Part print with two shaded views. Sizes in mm from the minimum x, y, z corner. Round coordinates to 2 decimals unless told otherwise and drop trailing zeros. Loops run counter-clockwise (first coordinate to the right, second up) from the corner with the lowest first, then second, coordinate; pieces in that order, holes last. Notation, with made-up numbers: M 49.5,48 L 55.5,48 A36 ccw 55.5,82 Z; hole C 40.5,54 d5. An arc over 180 degrees is marked long. Answer as CSV lines item,"result". Start each with the question number.
Item 1: Band-saw the part on C-C (z = 5.5). Give the cut face in (x, y).
Item 2: Band-saw the part on D-D (x = 6). Give the cut face in (y, z), and give its area (3 significant figures).
Item 3: Wall check: line 1 (X direction, y = 9.5, z = 51); line 2 (Z direction, x = 27.5, y = 10.5); line 3 (Y direction, x = 13, z = 11). Give the ranges that are in metal, low to high.
Item 4: Band-saw the part on B-B (y = 43). Give the cut face in (x, z), and give its area (3 significant figures).
Item 5: Mould opens along X. For the marked faces 1, 2 and 3 say: pulls with the +X half, pulls with the -X half, needs draft (parallel to the pull), parting line crosses it, or undercut.
Item 6: Drop flat-ended pins along their axis: pin 1 Ø5 at (x, z) = (12.5, 41.5) entering from -Y; pin 2 Ø6 at (x, y) = (15, 16) entering from -Z; pin 3 Ø3 at (x, z) = (9, 66) entering from -Y. Give the stop position or say it passes through.
Item 7: Band-saw the part on A-A (x = 60.5). Give the cut face in (y, z), and give its area (3 significant figures).
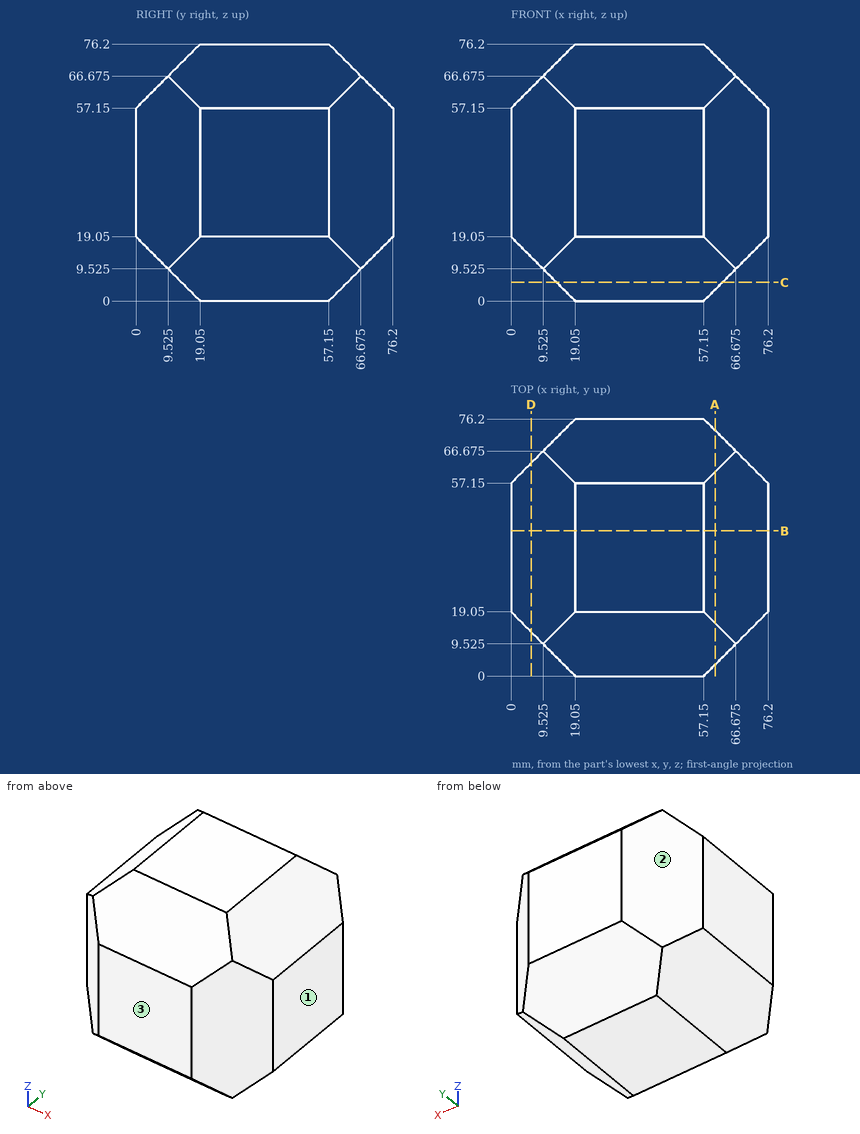
Answer block:
1,outline,"M 13.55,13.55 L 62.65,13.55 L 62.65,62.65 L 13.55,62.65 Z"
2,outline,"M 13.05,13.05 L 63.15,13.05 L 63.15,63.15 L 13.05,63.15 Z"
2,area,"2,510 mm^2"
3,line 1,"x = 9.55 to 66.65"
3,line 2,"z = 8.55 to 67.65"
3,line 3,"y = 8.05 to 68.15"
4,outline,"M 0,19.05 L 19.05,0 L 57.15,0 L 76.2,19.05 L 76.2,57.15 L 57.15,76.2 L 19.05,76.2 L 0,57.15 Z"
4,area,"5,080 mm^2"
5,face 1,"pulls with the +X half"
5,face 2,"pulls with the -X half"
5,face 3,"needs draft"
6,pin 1,"stops at y = 4.05"
6,pin 2,"stops at z = 1.49"
6,pin 3,"stops at y = 8.58"
7,outline,"M 3.35,15.7 L 15.7,3.35 L 60.5,3.35 L 72.85,15.7 L 72.85,60.5 L 60.5,72.85 L 15.7,72.85 L 3.35,60.5 Z"
7,area,"4,530 mm^2"
